```python
from build123d import *

# Parameters (mm, degrees)
BOSS_EXTRUDE2_DEPTH     = 7
CUT_EXTRUDE2_DEPTH      = 30.130224853
CUT_EXTRUDE2_DEPTH_BACK = 30.130224853
SKETCH3_R               = 2
BOSS_EXTRUDE3_DEPTH     = 36
SKETCH5_R               = 2
BOSS_EXTRUDE4_DEPTH     = 7
SKETCH13_W              = 49.8
SKETCH13_H              = 5
BOSS_EXTRUDE6_DEPTH     = 12.25
SKETCH15_W              = 49.8
SKETCH15_H              = 5
BOSS_EXTRUDE7_DEPTH     = 30
BOSS_EXTRUDE8_DEPTH     = 5
CUT_EXTRUDE3_DEPTH      = 150.404134049
CUT_EXTRUDE3_DEPTH_BACK = 150.404134049
SKETCH16_R              = 2.625
SKETCH16_R_2            = 1.5


with BuildPart() as part:
    # Sketch1 → Boss-Extrude2 (new body)
    with BuildSketch(Plane(origin=(0, 0, 0), x_dir=(1, 0, 0), z_dir=(0, 1, 0))):
        with BuildLine():
            Line((-24.9, 0), (-24.9, 13.4))
            Line((-24.9, 13.4), (24.9, 13.4))
            Line((24.9, 13.4), (24.9, 0))
            ThreePointArc((24.9, 0), (23.392904185, -4.800819919), (19.412411454, -7.878950407))
            Line((19.412411454, -7.878950407), (8.235013612, 1.5))
            ThreePointArc((8.235013612, 1.5), (11.116692467, 6.448255578), (16.5, 8.4))
            Line((16.5, 8.4), (-16.5, 8.4))
            ThreePointArc((-16.5, 8.4), (-11.116692467, 6.448255578), (-8.235013612, 1.5))
            Line((-8.235013612, 1.5), (-19.412411454, -7.878950407))
            ThreePointArc((-19.412411454, -7.878950407), (-23.392904185, -4.800819919), (-24.9, 0))
        make_face()
    extrude(amount=BOSS_EXTRUDE2_DEPTH)

    # Sketch3 → Cut-Extrude2 (cut, two sides: drawn at the far end of the back side and taken through both)
    with BuildSketch(Plane(origin=(0, 7, 0), x_dir=(1, 0, 0), z_dir=(0, 1, 0)).offset(-CUT_EXTRUDE2_DEPTH_BACK)):
        with Locations(Location((-16.5, 0, 0), (0, 0, 270))):
            Circle(SKETCH3_R)
        with Locations(Location((16.5, 0, 0), (0, 0, 270))):
            Circle(SKETCH3_R)
    extrude(amount=CUT_EXTRUDE2_DEPTH + CUT_EXTRUDE2_DEPTH_BACK, mode=Mode.SUBTRACT)

    # Sketch4 → Boss-Extrude3 (add)
    with BuildSketch(Plane(origin=(0, 7, 0), x_dir=(1, 0, 0), z_dir=(0, 1, 0))):
        Polygon((-24.9, 13.4), (-24.9, 0), (-20.9, 0), (-20.9, 8.4), (-16.5, 8.4), (16.5, 8.4), (20.9, 8.4), (20.9, 0), (24.9, 0), (24.9, 13.4), align=None)
    extrude(amount=BOSS_EXTRUDE3_DEPTH)

    # Sketch5 → Boss-Extrude4 (add)
    with BuildSketch(Plane(origin=(0, 43, 0), x_dir=(1, 0, 0), z_dir=(0, 1, 0))):
        with BuildLine():
            Line((-24.9, 13.4), (-24.9, 0))
            ThreePointArc((-24.9, 0), (-23.392904185, -4.800819919), (-19.412411454, -7.878950407))
            Line((-19.412411454, -7.878950407), (-8.235013612, 1.5))
            ThreePointArc((-8.235013612, 1.5), (-11.116692467, 6.448255578), (-16.5, 8.4))
            Line((-16.5, 8.4), (16.5, 8.4))
            ThreePointArc((16.5, 8.4), (11.116692467, 6.448255578), (8.235013612, 1.5))
            Line((8.235013612, 1.5), (19.412411454, -7.878950407))
            ThreePointArc((19.412411454, -7.878950407), (23.392904185, -4.800819919), (24.9, 0))
            Line((24.9, 0), (24.9, 13.4))
            Line((24.9, 13.4), (-24.9, 13.4))
        make_face()
        with Locations(Location((16.5, 0, 0), (0, 0, 270))):
            Circle(SKETCH5_R, mode=Mode.SUBTRACT)
        with Locations(Location((-16.5, 0, 0), (0, 0, 270))):
            Circle(SKETCH5_R, mode=Mode.SUBTRACT)
    extrude(amount=BOSS_EXTRUDE4_DEPTH)

    # Sketch13 → Boss-Extrude6 (add)
    with BuildSketch(Plane(origin=(0, 50, 0), x_dir=(1, 0, 0), z_dir=(0, 1, 0))):
        with Locations((0, 10.9)):
            Rectangle(SKETCH13_W, SKETCH13_H)
    extrude(amount=BOSS_EXTRUDE6_DEPTH)

    # Sketch15 → Boss-Extrude7 (add)
    with BuildSketch(Plane.XZ):
        with Locations((0, -10.9)):
            Rectangle(SKETCH15_W, SKETCH15_H)
    extrude(amount=BOSS_EXTRUDE7_DEPTH)

    # Sketch12 → Boss-Extrude8 (add)
    with BuildSketch(Plane(origin=(0, 0, -13.4), x_dir=(-1, 0, 0), z_dir=(0, 0, -1))):
        Polygon((24.9, -30), (24.9, -41.497235918), (93.105904535, -57.243809722), (79.608841274, -115.706013609), (-67.628165204, -81.713672257), (-54.131101944, -23.25146837), (-24.9, -30), align=None)
    extrude(amount=-BOSS_EXTRUDE8_DEPTH)

    # Sketch16 → Cut-Extrude3 (cut, two sides: drawn at the far end of the back side and taken through both)
    with BuildSketch(Plane.XY.offset(-8.4).offset(-CUT_EXTRUDE3_DEPTH_BACK)):
        with Locations((42.889816787, -41.241285157)):
            Circle(SKETCH16_R)
        with Locations((50.684777305, -39.441676722)):
            Circle(SKETCH16_R_2)
        with Locations((44.689425222, -49.036245675)):
            Circle(SKETCH16_R_2)
        with Locations((35.094856269, -43.040893591)):
            Circle(SKETCH16_R_2)
        with Locations((41.090208352, -33.446324638)):
            Circle(SKETCH16_R_2)
        with Locations((-82.911048266, -70.284703313)):
            Circle(SKETCH16_R_2)
        with Locations((-76.915696183, -60.69013436)):
            Circle(SKETCH16_R_2)
        with Locations((-67.32112723, -66.685486444)):
            Circle(SKETCH16_R_2)
        with Locations((-73.316479313, -76.280055397)):
            Circle(SKETCH16_R_2)
        with Locations((-75.116087748, -68.485094879)):
            Circle(SKETCH16_R)
        with Locations(Location((47.838739983, -62.677426582, 0), (0, 0, 180))):
            Circle(SKETCH16_R_2)
        with Locations(Location((57.433308936, -68.672778665, 0), (0, 0, 180))):
            Circle(SKETCH16_R_2)
        with Locations(Location((51.437956852, -78.267347618, 0), (0, 0, 180))):
            Circle(SKETCH16_R_2)
        with Locations(Location((49.638348417, -70.4723871, 0), (0, 0, 180))):
            Circle(SKETCH16_R)
        with Locations(Location((41.843387899, -72.271995535, 0), (0, 0, 180))):
            Circle(SKETCH16_R_2)
        with Locations(Location((-70.167164552, -89.921236304, 0), (0, 0, 180))):
            Circle(SKETCH16_R_2)
        with Locations(Location((-68.367556118, -97.716196822, 0), (0, 0, 180))):
            Circle(SKETCH16_R)
        with Locations(Location((-76.162516636, -99.515805257, 0), (0, 0, 180))):
            Circle(SKETCH16_R_2)
        with Locations(Location((-66.567947683, -105.511157341, 0), (0, 0, 180))):
            Circle(SKETCH16_R_2)
        with Locations(Location((-60.572595599, -95.916588388, 0), (0, 0, 180))):
            Circle(SKETCH16_R_2)
    extrude(amount=CUT_EXTRUDE3_DEPTH + CUT_EXTRUDE3_DEPTH_BACK, mode=Mode.SUBTRACT)


solid = part.part
```
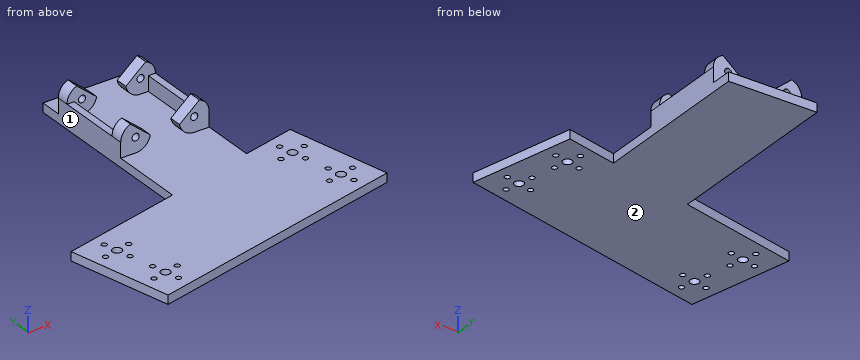
For this review, take the finished solid that the model builds, in its own axes (mm). Face numbers are marked on the shaded views. A direction names the side the tool comes from. Round coordinates to 2 decimals unless told otherwise and drop trailing zeros. Order: outer loops, then holes, each group sorted by start corner. A loop starts at its lowest first (then second) coordinate and runs counter-clockwise, first axis right, second up. Notation, with made-up numbers: (37, -15) -> (53, -15) arc R10 cw to (53, -4) -> close; hole circle Ø9 at (19, 2.5). An arc over 180 degrees is marked (long way). Use a Markdown table: item, result.
Item 1: Take a section at B-B (y = 33.5). State the section outline as (x, z) points.
Resolved:
| item | result |
|---|---|
| outline | (-24.9, -13.4) -> (24.9, -13.4) -> (24.9, 0) -> (20.9, 0) -> (20.9, -8.4) -> (-20.9, -8.4) -> (-20.9, 0) -> (-24.9, 0) -> close |
Item 2: Machinability: for the marked faces 1 and 2, which of the approach directions +Z, -Z, +X, -X, +Y, -Y give a long, thin tool a straight path to every point of the face, cutting with its end or side? Answer none if there is none.
Resolved:
| item | result |
|---|---|
| face 1 | +Z, -Z, -X, +Y |
| face 2 | -Z, +X, -X, +Y, -Y |
Item 3: For pin 1 (2.5 mm diameter, centred on x = -67.32, y = -66.69, fed in from -Z); pin 2 (10 mm diameter, centred on y = -84.5, z = -10.5, fed in from -X); pin 3 (6 mm diameter, centred on x = 25.5, z = 1.5, fed in from +Y); pin 4 (5 mm diameter, centred on x = 50.68, y = -39.44, fed in from -Z), all flat-tipped, find the tip position at first contact; note any pin that passes through.
Resolved:
| item | result |
|---|---|
| pin 1 | passes through |
| pin 2 | stops at x = -87.97 |
| pin 3 | stops at y = 50 |
| pin 4 | stops at z = -13.4 |
Item 4: Take a section at D-D (x = -1). State the section outline as (y, z) points.
Resolved:
| item | result |
|---|---|
| outline | (-97.56, -13.4) -> (62.25, -13.4) -> (62.25, -8.4) -> (-97.56, -8.4) -> close |
Item 5: Take a section at C-C (x = -51). State the section outline as (y, z) points, plus the area to 3 significant figures.
Resolved:
| item | result |
|---|---|
| outline | (-109.1, -13.4) -> (-47.52, -13.4) -> (-47.52, -8.4) -> (-109.1, -8.4) -> close |
| area | 308 mm² |
Item 6: For line 1 along Y through (x, z) = (-23, 1.25); line 2 along Z through (x, y) = (5, -69); line 3 along Y through (x, z) = (22.5, -6.5), list the stretches that pass through material, from the lowest coordinate up. Write a range as [from, to].
Resolved:
| item | result |
|---|---|
| line 1 | y = [0, 7], [43, 50] |
| line 2 | z = [-13.4, -8.4] |
| line 3 | y = [0, 50] |
Item 7: Take a section at A-A (z = 5.25). State the section outline as (x, y) points.
Resolved:
| item | result |
|---|---|
| outline | (-23.06, 0) -> (-16.28, 0) -> (-16.28, 7) -> (-23.06, 7) -> close; (-23.06, 43) -> (-16.28, 43) -> (-16.28, 50) -> (-23.06, 50) -> close; (16.28, 0) -> (23.06, 0) -> (23.06, 7) -> (16.28, 7) -> close; (16.28, 43) -> (23.06, 43) -> (23.06, 50) -> (16.28, 50) -> close |
